The drawing under review shows one solid part. Ordinate dimensions are in mm from its lowest x, y, z. Give positions to 0.01 mm unless a question says otherwise; leave off trailing zeros. Write each loop counter-clockwise with the first axis right and the second up, starting at its lowest first coordinate (ties: lowest second). Pieces come first, ordered by that corner, then holes.
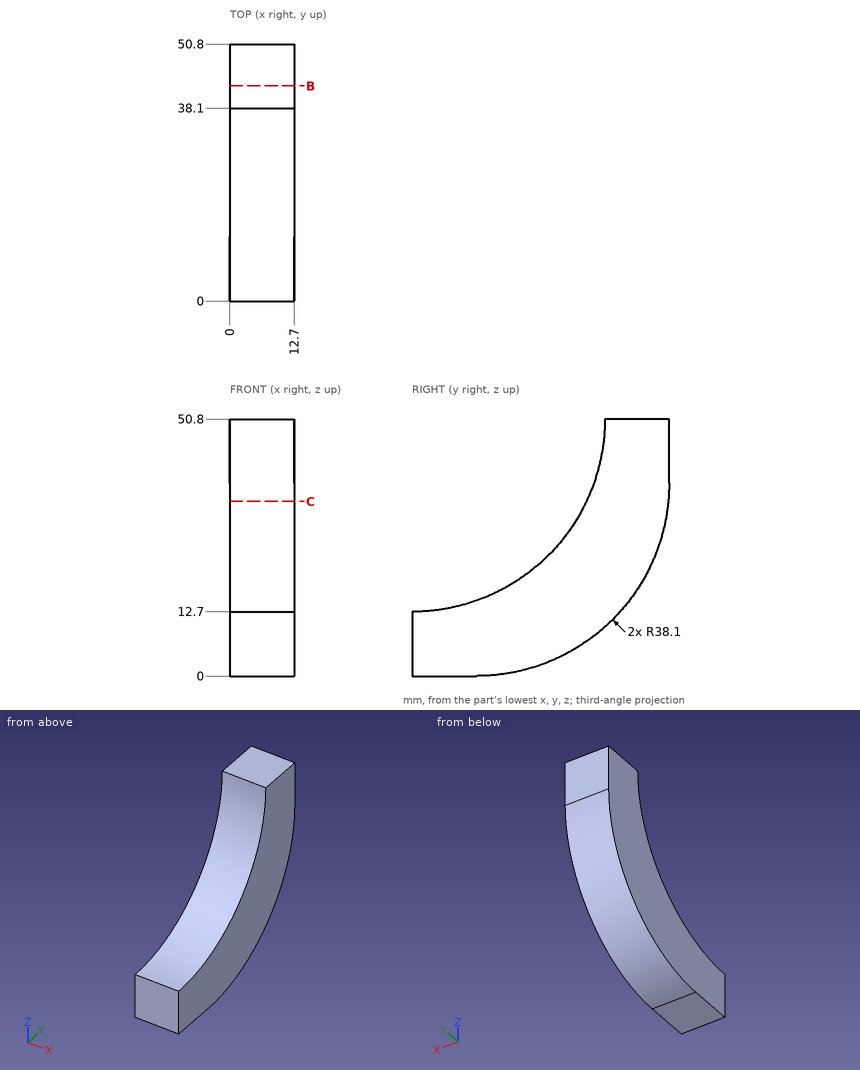
1) To check wall thickness, follow probe 1 along Y at (x, z) = (9.25, 21); probe 2 along Y at (x, z) = (5.75, 23); probe 3 along Z at (x, y) = (8.5, 7.5). State the ranges of each line that lie inside material, in increasing order.
2) Consider section B-B, the plane y = 42.5. Give the boundary of the cut face in (x, z), then the cut area to 3 significant figures.
3) Consider section C-C, the plane z = 34.5. Give the boundary of the cut face in (x, y), then the cut area to 3 significant figures.
4) Insertion check: pin 1 (1.5 mm diameter, centred on x = 5.5, z = 34, fed in from -Y); pin 2 (1.5 mm diameter, centred on y = 41, z = 28, fed in from -X); pin 3 (3 mm diameter, centred on x = 7, y = 24.5, fed in from +Z); pin 4 (5 mm diameter, centred on x = 9.5, y = 41, fed in from -Z) (1 decimal). Each pin has a flat end and moves straight along its axis. Give the tip position at first contact, or say it passes through.
Answer block:
1. probe 1: y = 23.74 to 46.75
1. probe 2: y = 26.05 to 47.68
1. probe 3: z = 0 to 13.45
2. outline: (0, 14.36) - (12.7, 14.36) - (12.7, 50.8) - (0, 50.8) - close
2. area: 463 mm2
3. outline: (0, 34.44) - (12.7, 34.44) - (12.7, 50.63) - (0, 50.63) - close
3. area: 206 mm2
4. pin 1: stops at y = 33.82
4. pin 2: stops at x = 0
4. pin 3: stops at z = 22.95
4. pin 4: stops at z = 10.1
